from build123d import *

# Parameters (mm, degrees)
CUT_EXTRUDE_1_DEPTH      = 67.373183556
CUT_EXTRUDE_1_DEPTH_BACK = 67.373183556


# Read off the part's stored shape, not the designer's step: Поверхность-Сшить1
with BuildPart() as part:
    # Knit 1 outline → Knit 1 (revolve)
    with BuildSketch(Plane.XY):
        with BuildLine():
            Line((0, 0), (0, -40))
            Line((0, -40), (20, -40))
            ThreePointArc((20, -40), (24.059865396, -20.194983175), (25, 0))
            Line((25, 0), (0, 0))
        make_face()
    revolve(axis=Axis((0, 0, 0), (0, 1, 0)))

    # По траектории1: sweep along a path in Эскиз3
    with BuildLine(Plane(origin=(0, 0, 0), x_dir=(0, 0, -1), z_dir=(1, 0, 0))) as sweep_1_path:
        ThreePointArc((32.759858657, 0), (29.894665497, -26.609940967), (21.430435325, -52))
    # Эскиз2 → По траектории1 (sweep)
    with BuildSketch(Plane(origin=(0, 0, 0), x_dir=(1, 0, 0), z_dir=(0, 1, 0))):
        with BuildLine():
            Line((-15, 0), (15, 0))
            Line((15, 0), (11, 32))
            ThreePointArc((11, 32), (0, 32.759858657), (-11, 32))
            Line((-11, 32), (-15, 0))
        make_face()
    sweep(path=sweep_1_path.line)

    # Эскиз4 → Вырез-Вытянуть1 (cut, two sides: drawn at the far end of the back side and taken through both)
    with BuildSketch(Plane.XY.offset(-CUT_EXTRUDE_1_DEPTH_BACK)):
        with BuildLine():
            Line((145.597430233, 60.060046505), (31.407892686, -38.452179183))
            ThreePointArc((31.407892686, -38.452179183), (-1.252964611, -50.593647771), (-33.913821908, -38.452179183))
            Line((-33.913821908, -38.452179183), (-148.103359455, 60.060046505))
            Line((-148.103359455, 60.060046505), (-148.103359455, -241.561631066))
            Line((-148.103359455, -241.561631066), (145.597430233, -241.561631066))
            Line((145.597430233, -241.561631066), (145.597430233, 60.060046505))
        make_face()
    extrude(amount=CUT_EXTRUDE_1_DEPTH + CUT_EXTRUDE_1_DEPTH_BACK, mode=Mode.SUBTRACT)


solid = part.part
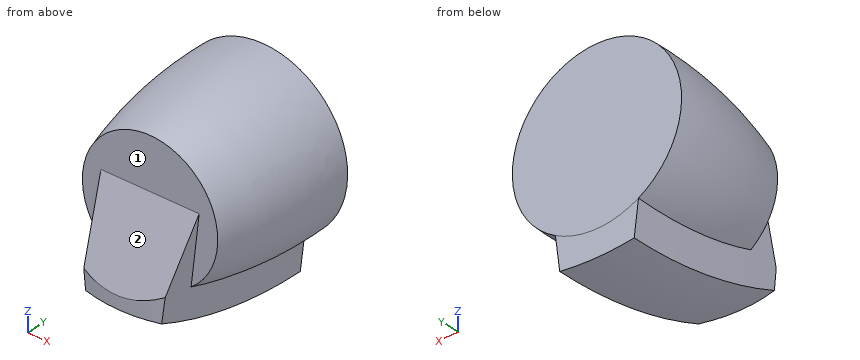
Input: part model. Units: mm. Frame: model coordinates. Face numbers are marked on the shaded views. A direction names the side the tool comes from. Coordinates: 2 decimals unless noted, no trailing zeros. Answer as CSV lines item,"result".
1. Access query for the marked faces 1 and 2. Directions: +Z, -Z, +X, -X, +Y, -Y. A direction counts if a zero-diameter tool reaches every point of the face in a straight line with its end or side. Return the directions, or none.
Reported:
face 1,"-Y"
face 2,"+Z, +X, -X, -Y"
2. First-contact query: P1, Ø2, axis at x = 14.5, y = -41.5, coming from the +Z side; P2, Ø2, axis at x = -17.5, y = -38, coming from the +Z side; P3, Ø10, axis at y = -7.5, z = -23.5, coming from the -X side. Flat tips, straight axial feed; report the tip coordinate or a pass-through.
Reported:
P1,"z = 3.69"
P2,"z = 12.34"
P3,"x = -16.85"
3. Material intervals for line 1 (Y direction, x = -4.5, z = 11.5); line 2 (Y direction, x = 12, z = -7); line 3 (Z direction, x = -6, y = -30.5), sorted ascending. Write a range as from..to.
Reported:
line 1,"-40..0"
line 2,"-45.4..0"
line 3,"-28.75..21.53"
